Solid Edge part; units mm, degrees
sketch "Sketch1" plane through (0, 0, 0) normal (0, 0, 1) x (1, 0, 0)
  line L0 (0, 0) -> (100, 0)
  line L1 (100, 0) -> (100, 100)
  line L2 (100, 100) -> (0, 100)
  line L3 (0, 100) -> (0, 0)
extrude "Protrusion1" add sketch "Sketch1" along normal blind 15
hole "Hole_1" at (80, 80, 15) direction (0, 0, -1) diameter 10 end through all
hole "Hole1" at (80, 20, 15) direction (0, 0, -1) diameter 10 end through all
hole "Hole2" at (20, 20, 15) direction (0, 0, -1) diameter 10 end through all
hole "Hole3" at (20, 80, 15) direction (0, 0, -1) diameter 10 end through all
sketch "Sketch2" plane through (50, 50, 0) normal (0, 0, -1) x (0, -1, 0)
  line L0 (-20, 20) -> (20, 20)
  line L1 (20, 20) -> (20, -20)
  line L2 (20, -20) -> (-20, -20)
  line L3 (-20, -20) -> (-20, 20)
extrude "Cutout1" cut sketch "Sketch2" against normal through all
fillet "Round_2" radius 6 4 edges at (30, 70, 7.5) (70, 70, 7.5) (70, 30, 7.5) (30, 30, 7.5)
properties part number "1000"
Model file for the job. Use its own axes, mm. A direction names the side the tool comes from. Give positions to 0.01 mm unless a question says otherwise; leave off trailing zeros. Write each loop counter-clockwise with the first axis right and the second up, starting at its lowest first coordinate (ties: lowest second). Pieces come first, ordered by that corner, then holes. Notation, with made-up numbers: (-9.5, 6) -> (31.5, 6) arc R25 cw to (31.5, 37) -> close; hole circle Ø7 at (19, -3.75). An arc over 180 degrees is marked (long way). Use CSV: the item, a comma, the result in double quotes. Start each with the question number.
1) Two-plate mould, pull along X, no slides. Class faces 1 (the flat face through (27, 51, 15)), 2 (the cylindrical face through (31.711, 31.804, 7.605)), 3 (the flat face through (0, 51, 7)), 4 (the flat face through (30, 50, 7)): released by +X, released by -X, zero draft, split by the parting line, or undercut.
2) Cut at D-D on z = 8.5. List the corners of the cut face in (x, y), plus the area to 3 significant figures.
3) Pin check, flat tips, straight feed: P1, Ø8, axis at x = 80, y = 20, coming from the -Z side (3 decimals); P2, Ø5, axis at x = 43, z = 5, coming from the -Y side. Stop position of each tip, or through.
4) Cut at B-B on y = 38.5. List the corners of the cut face in (x, z), plus the area to 3 significant figures.
5) Drill centre lines: L1, parallel to X at y = 20, z = 9; L2, parallel to Y at x = 64.5, z = 3.25. Where is each one in solid material? Low to high.
6) Cut at A-A on y = 20. List the corners of the cut face in (x, z), plus the area to 3 significant figures.
7) Tool access for faces 5 (the flat face through (27, 51, 0)), 6 (the flat face through (50, 30, 7)): list every direction of +Z, -Z, +X, -X, +Y, -Y with a clear straight run to the whole face (end or side of a thin tool).
Final values:
1,face 1,"zero draft"
1,face 2,"undercut"
1,face 3,"released by -X"
1,face 4,"undercut"
2,outline,"(0, 0) -> (100, 0) -> (100, 100) -> (0, 100) -> close; hole circle Ø10 at (20, 20); hole circle Ø10 at (20, 80); hole (30, 36) arc R6 ccw to (36, 30) -> (64, 30) arc R6 ccw to (70, 36) -> (70, 64) arc R6 ccw to (64, 70) -> (36, 70) arc R6 ccw to (30, 64) -> close; hole circle Ø10 at (80, 20); hole circle Ø10 at (80, 80)"
2,area,"8,120 mm2"
3,P1,"passes through"
3,P2,"stops at y = 0"
4,outline,"(0, 0) -> (30, 0) -> (30, 15) -> (0, 15) -> close; (70, 0) -> (100, 0) -> (100, 15) -> (70, 15) -> close"
4,area,"900 mm2"
5,L1,"x = 0 to 15, 25 to 75, 85 to 100"
5,L2,"y = 0 to 30.02, 69.98 to 100"
6,outline,"(0, 0) -> (15, 0) -> (15, 15) -> (0, 15) -> close; (25, 0) -> (75, 0) -> (75, 15) -> (25, 15) -> close; (85, 0) -> (100, 0) -> (100, 15) -> (85, 15) -> close"
6,area,"1,200 mm2"
7,face 5,"-Z, +X, -X, +Y, -Y"
7,face 6,"+Z, -Z"
